Model file for the job. Use its own axes, mm. A direction names the side the tool comes from. Give positions to 0.01 mm unless a question says otherwise; leave off trailing zeros. Loops run counter-clockwise (first coordinate to the right, second up) from the corner with the lowest first, then second, coordinate; pieces in that order, holes last. Notation, with made-up numbers: M 72.5,45.25 L 128.5,45.25 A22 ccw 128.5,57.25 Z; hole C 23.25,-3 d1. An arc over 180 degrees is marked long. Answer in a Markdown table with one row per item.
Autodesk Inventor part; units mm, degrees
ref_plane "Work Plane1" through (0, 9, 0) normal (0, 1, 0) x (1, 0, 0)
ref_plane "YZ Plane" through (0, 0, 0) normal (1, 0, 0) x (0, 1, 0)
ref_plane "XZ Plane" through (0, 0, 0) normal (0, 1, 0) x (-1, 0, 0)
sketch "Sketch1" plane through (0, 0, 0) normal (0, 1, 0) x (-1, 0, 0)
  circle A0 centre (0, 0) radius 4
  dimension "d0" = 8
extrude "Extrusion1" add sketch "Sketch1" along normal blind 4.5
ref_plane "Work Plane1" through (0, 9, 0) normal (0, 1, 0) x (1, 0, 0)
sketch "Sketch2" plane through (0, 9, 0) normal (0, 1, 0) x (1, 0, 0)
  circle A0 centre (0, 0) radius 1.75
  dimension "d4" = 3.5
loft "Loft1" add profiles "Sketch2" section 1 edges at (4, 4.5, 0)
sketch "Sketch3" plane through (0, 9, 0) normal (0, 1, 0) x (1, 0, 0)
  circle A0 centre (0, 0) radius 1
  dimension "d9" = 2
sketch "Sketch4" plane through (0, 0, 0) normal (0, -1, 0) x (1, 0, 0)
  circle A0 centre (0, 0) radius 1.75
  line L0 (6.5, 0) -> (3.25, -5.6292)
  line L1 (3.25, -5.6292) -> (-3.25, -5.6292)
  line L2 (-3.25, -5.6292) -> (-6.5, 0)
  line L3 (-6.5, 0) -> (-3.25, 5.6292)
  line L4 (-3.25, 5.6292) -> (3.25, 5.6292)
  line L5 (3.25, 5.6292) -> (6.5, 0)
extrude "Extrusion2" add sketch "Sketch4" along normal blind 5.5
sketch "Sketch5" plane through (0, -5.5, 0) normal (0, -1, 0) x (1, 0, 0)
  circle A0 centre (0, 0) radius 7.5
  dimension "d12" = 15
extrude "Extrusion3" add sketch "Sketch5" along normal blind 2
sketch "Sketch6" plane through (0, -7.5, 0) normal (0, -1, 0) x (1, 0, 0)
  circle A0 centre (0, 0) radius 5
  dimension "d15" = 10
extrude "Extrusion4" add sketch "Sketch6" along normal blind 14
thread "Thread1"
extrude "Extrusion5" cut sketch "Sketch3" against normal up to surface (30.5 mm away)
properties part number "ZKE-Term-Sprung-17.5mm"
(1) Which spindle directions (+Z, -Z, +X, -X, +Y, -Y) get a long thin tool onto all of the face, cutting with end or side? Do faces 4 (the flat face through (-5, -5.5, -3)), 5 (the cylindrical face through (-1.08, -14.4, 4.88)), 6 (the flat face through (0, -3, -5.629)), 7 (the cylindrical face through (1.617, -2.712, 0.67)), 8 (the flat face through (-4.852, -2.712, -2.854)). Say none if no direction does.
Established:
| item | result |
|---|---|
| face 4 | +Y |
| face 5 | -Y |
| face 6 | -Z, +X, -X, +Y |
| face 7 | none |
| face 8 | -Z, -X, +Y |
(2) Saw through at B-B, the plane y = -18. Give the cut face in (x, z), and give its area (3 significant figures).
Established:
| item | result |
|---|---|
| outline | C 0,0 d10; hole C 0,0 d2 |
| area | 75.4 mm2 |
(3) Mould opens along X. For faces 1 (the flat face through (1, -5.5, -1)), 2 (the flat face through (0, -3, 5.629)), 3 (the flat face through (-4.898, -2.712, 2.775)) say: pulls with the +X half, pulls with the -X half, needs draft (parallel to the pull), parting line crosses it, or undercut.
Established:
| item | result |
|---|---|
| face 1 | undercut |
| face 2 | needs draft |
| face 3 | pulls with the -X half |
(4) Flat gauge pins, fed straight in: P1, Ø8, axis at y = -12.5, z = -5.5, coming from the -X side; P2, Ø2, axis at y = -15, z = 4, coming from the -X side; P3, Ø6, axis at x = 1.5, y = -1.5, coming from the +Z side; P4, Ø1.6, axis at x = 0, z = 0, coming from the +Y side. Where does each tip first touch, or does it go through?
Established:
| item | result |
|---|---|
| P1 | stops at x = -4.77 |
| P2 | stops at x = -4 |
| P3 | stops at z = 5.63 |
| P4 | passes through |
(5) Wall check: L1, parallel to X at y = 2.5, z = 0; L2, parallel to Z at x = 0, y = -12.75; L3, parallel to Z at x = 0, y = -2.95. Give the ranges that are in metal, low to high.
Established:
| item | result |
|---|---|
| L1 | x = -4 to -1, 1 to 4 |
| L2 | z = -5 to -1, 1 to 5 |
| L3 | z = -5.63 to -1.75, 1.75 to 5.63 |
(6) Saw through at C-C, the plane x = 6. Give the cut face in (y, z).
Established:
| item | result |
|---|---|
| outline | M -7.5,-4.5 L -5.5,-4.5 L -5.5,-0.87 L 0,-0.87 L 0,0.87 L -5.5,0.87 L -5.5,4.5 L -7.5,4.5 Z |
